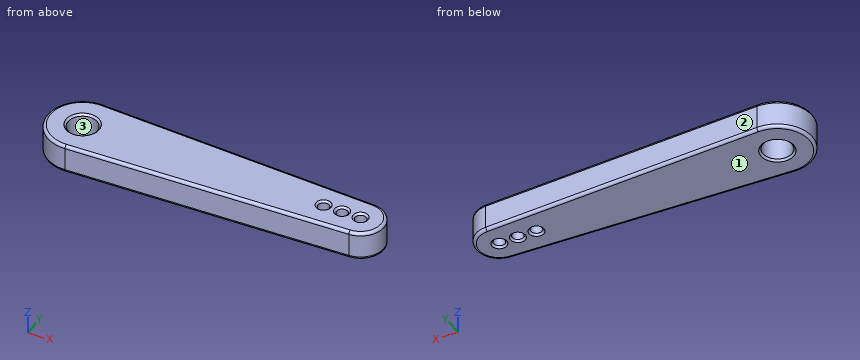
```python
from build123d import *

# Parameters (mm, degrees)
SKETCH1_R           = 3.96875
SKETCH1_R_2         = 1.524
BOSS_EXTRUDE1_DEPTH = 7.9375
FILLET2_R           = 0.79375
CHAMFER1_SIZE       = 0.529166667


with BuildPart() as part:
    # Sketch1 → Boss-Extrude1 (new body)
    with BuildSketch(Plane.XY):
        with BuildLine():
            Line((-37.703125, 9.516728179), (38.364583333, 6.344485453))
            ThreePointArc((38.364583333, 6.344485453), (44.45, 0), (38.364583333, -6.344485453))
            Line((38.364583333, -6.344485453), (-37.703125, -9.516728179))
            ThreePointArc((-37.703125, -9.516728179), (-47.625, 0), (-37.703125, 9.516728179))
        make_face()
        with Locations((-38.1, 0)):
            Circle(SKETCH1_R, mode=Mode.SUBTRACT)
        with Locations((38.1, 0)):
            Circle(SKETCH1_R_2, mode=Mode.SUBTRACT)
        with Locations((33.02, 0)):
            Circle(SKETCH1_R_2, mode=Mode.SUBTRACT)
        with Locations((27.94, 0)):
            Circle(SKETCH1_R_2, mode=Mode.SUBTRACT)
    extrude(amount=BOSS_EXTRUDE1_DEPTH)

    # Fillet2
    fillet2_edges = [part.edges().sort_by_distance(p)[0] for p in [
        (44.45, 0, 7.9375),
        (0.330729167, 7.930606816, 7.9375),
        (-47.625, 0, 7.9375),
        (0.330729167, 7.930606816, 0),
        (44.45, 0, 0),
        (0.330729167, -7.930606816, 0),
        (-47.625, 0, 0),
        (0.330729167, -7.930606816, 7.9375),
    ]]
    fillet(fillet2_edges, radius=FILLET2_R)

    # Chamfer1
    chamfer1_edges = [part.edges().sort_by_distance(p)[0] for p in [
        (-42.06875, 0, 0),
        (-42.06875, 0, 7.9375),
        (36.576, 0, 0),
        (36.576, 0, 7.9375),
        (31.496, 0, 0),
        (31.496, 0, 7.9375),
        (26.416, 0, 0),
        (26.416, 0, 7.9375),
    ]]
    chamfer(chamfer1_edges, length=CHAMFER1_SIZE)


solid = part.part
```
The listing builds one solid part. Answer for the finished solid, in the listing's coordinates (mm). Face numbers are marked on the shaded views. Coordinates: 2 decimals unless noted, no trailing zeros. Return JSON: item names as keys, results as strings. Group by question number.
1. Given pin 1 (2 mm diameter, centred on x = -22.5, z = 3.5, fed in from -Y); pin 2 (2 mm diameter, centred on x = -24, z = 6, fed in from -Y); pin 3 (4 mm diameter, centred on x = 38.1, y = 0, fed in from +Z); pin 4 (6.5 mm diameter, centred on x = -38.1, y = 0, fed in from +Z), each flat-ended and moving along its own axis, determine where each tip first touches the part or whether it passes through.
2. Determine the mould class of the marked faces 1, 2 and 3 for opening direction X: released by +X, released by -X, zero draft, split by the parting line, or undercut.
3. A cutting plane is placed at A-A, the plane z = 6. Give the number of separate pieces and of enclosed holes in the cut face, plus the area to 3 significant figures.
4. Straight lines are drawn through the part: L1, parallel to X at y = 1, z = 5.25; L2, parallel to X at y = -1.25, z = 2.5; L3, parallel to Y at x = 38, z = 6.5. For each, find the intervals that lie inside material, in ascending order.
Ans:
{
 "1": {"pin 1": "y = -8.92", "pin 2": "y = -8.99", "pin 3": "z = 7.88", "pin 4": "through"},
 "2": {"face 1": "zero draft", "face 2": "released by +X", "face 3": "undercut"},
 "3": {"separate pieces": "1", "enclosed holes": "4", "area": "1,350 mm²"},
 "4": {"L1": "-47.57 to -41.94, -34.26 to 26.79, 29.09 to 31.87, 34.17 to 36.95, 39.25 to 44.37", "L2": "-47.54 to -41.87, -34.33 to 27.07, 28.81 to 32.15, 33.89 to 37.23, 38.97 to 44.33", "L3": "-6.36 to -1.52, 1.52 to 6.36"}
}
